Can you work these out from the model? Positions are in its coordinate system, mm. A direction names the side the tool comes from. Round coordinates to 2 decimals unless told otherwise and drop trailing zeros. Write each loop counter-clockwise with the first axis right and the second up, starting at its lowest first coordinate (ties: lowest second). Pieces come first, ordered by that corner, then holes.
Q1. For faces 1 (the flat face through (-0.785, -2.567, -3.972)), 2 (the flat face through (1.831, -1.964, -3.972)), 3 (the flat face through (3, 1, -2)), 4 (the flat face through (2.616, 0.604, -3.972)), which set-ups out of +Z, -Z, +X, -X, +Y, -Y let a thin tool reach every point of the face, with its end or its side?
Q2. I'm going to push flat-ended pins straight in: pin 1 Ø2.5 at (x, y) = (2.23, 9.75) entering from -Z; pin 2 Ø3 at (x, y) = (-5, 1.5) entering from -Z; pin 3 Ø5 at (x, y) = (9.01, -4.34) entering from -Z. Where does each tip first touch, or does it pass through?
Q3. If we section it at D-D (x = -1): Please give me the cut outline in (y, z).
Q4. If we section it at C-C (z = -3.5): Please give me the cut outline in (x, y), plus the area to 3 significant figures.
Q5. If we section it at A-A (x = -10): Please give me the cut outline in (y, z).
Q6. Please list where these lines run through material, in increasing order: line 1 along Z through (x, y) = (11, -5.75); line 2 along Y through (x, z) = (-10, 0.25); line 3 along Y through (x, z) = (-0.25, 0.25).
Q7. We'd pull the mould along Y, two halves only. Please class faces 5 (the cylindrical face through (11.923, 3.755, 0.74)), 6 (the flat face through (-3, 3, 0)), 7 (the cylindrical face through (7.9, 5.35, 0.74)), 8 (the cylindrical face through (1.9, -11.214, 0.74)): +Y half, -Y half, draft (parallel to the pull), parting line (faces both ways), or undercut.
Q8. If we section it at B-B (y = 0): Please give me the cut outline in (x, z).
from build123d import *

# Parameters (mm, degrees)
F0_R     = 12.5
F0_R_2   = 1.5
F0_R_3   = 4
F1_DEPTH = 1.5
F2_DEPTH = 2
F4_DEPTH = 4


with BuildPart() as f1:
    # F0 (on Top) → F1 (new body)
    with BuildSketch(Plane.XY):
        Circle(F0_R)
        with Locations((-6.234898, -7.818315)):
            Circle(F0_R_2, mode=Mode.SUBTRACT)
        with Locations((2.225209, -9.749279)):
            Circle(F0_R_2, mode=Mode.SUBTRACT)
        with Locations((9.009689, -4.338837)):
            Circle(F0_R_2, mode=Mode.SUBTRACT)
        with Locations((-10, 0)):
            Circle(F0_R_2, mode=Mode.SUBTRACT)
        with Locations((-6.234898, 7.818315)):
            Circle(F0_R_2, mode=Mode.SUBTRACT)
        Circle(F0_R_3, mode=Mode.SUBTRACT)
        with Locations((9.009689, 4.338837)):
            Circle(F0_R_2, mode=Mode.SUBTRACT)
        with Locations((2.225209, 9.749279)):
            Circle(F0_R_2, mode=Mode.SUBTRACT)
        Circle(F0_R_3)
    extrude(amount=F1_DEPTH)

    # F0 (on Top) → F2 (join)
    with BuildSketch(Plane.XY):
        Circle(F0_R_3)
    extrude(amount=-F2_DEPTH)

    # F3 (on face) → F4 (join)
    with BuildSketch(Plane(origin=(0, 0, -2), x_dir=(1, 0, 0), z_dir=(0, 0, -1))):
        Polygon((-0.672768, -3.026117), (2.28431, -2.095692), (2.957078, 0.930425), (0.672768, 3.026117), (-2.28431, 2.095692), (-2.957078, -0.930425), align=None)
    extrude(amount=F4_DEPTH)


solid = f1.part
A:
1. face 1: -Z, -X, -Y
1. face 2: -Z, +X, -Y
1. face 3: -Z
1. face 4: -Z, +X, +Y
2. pin 1: passes through
2. pin 2: stops at z = -2
2. pin 3: stops at z = 0
3. outline: (-12.46, 0) - (-3.87, 0) - (-3.87, -2) - (-2.5, -2) - (-2.5, -6) - (2.73, -6) - (2.73, -2) - (3.87, -2) - (3.87, 0) - (12.46, 0) - (12.46, 1.5) - (-12.46, 1.5) - close
4. outline: (-2.96, 0.93) - (-2.28, -2.1) - (0.67, -3.03) - (2.96, -0.93) - (2.28, 2.1) - (-0.67, 3.03) - close
4. area: 25.0 mm2
5. outline: (-7.5, 0) - (-1.5, 0) - (-1.5, 1.5) - (-7.5, 1.5) - close; (1.5, 0) - (7.5, 0) - (7.5, 1.5) - (1.5, 1.5) - close
6. line 1: z = 0 to 1.5
6. line 2: y = -7.5 to -1.5, 1.5 to 7.5
6. line 3: y = -12.5 to 12.5
7. face 5: parting line
7. face 6: draft
7. face 7: undercut
7. face 8: undercut
8. outline: (-12.5, 0) - (-11.5, 0) - (-11.5, 1.5) - (-12.5, 1.5) - close; (-8.5, 0) - (-4, 0) - (-4, -2) - (-2.75, -2) - (-2.75, -6) - (2.75, -6) - (2.75, -2) - (4, -2) - (4, 0) - (12.5, 0) - (12.5, 1.5) - (-8.5, 1.5) - close
